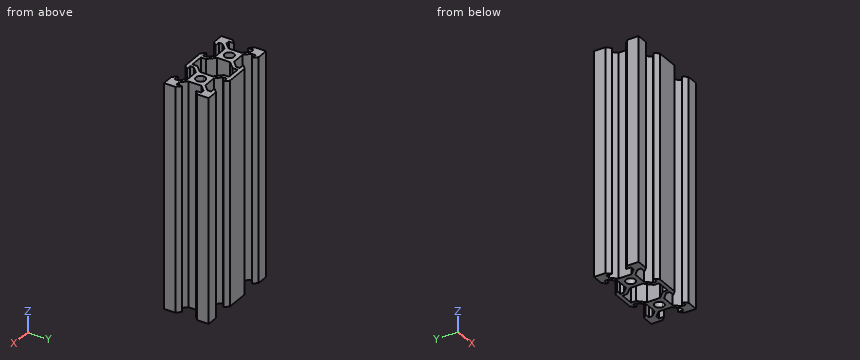
```python
from build123d import *

# Parameters (mm, degrees)
PAD_DEPTH            = 100
PAD_MIRRORED_2_DEPTH = 100


with BuildPart() as part:
    # Sketch → Pad (new body)
    with BuildSketch(Plane.XY):
        with BuildLine():
            Line((0, 10), (5.1, 10))
            Line((5.1, 10), (6.9, 8.2))
            Line((6.9, 8.2), (4.5, 8.2))
            Line((4.5, 8.2), (4.5, 6.56066))
            Line((4.5, 6.56066), (7.06066, 4))
            Line((7.06066, 4), (12.93934, 4))
            Line((12.93934, 4), (15.5, 6.56066))
            Line((15.5, 6.56066), (15.5, 8.2))
            Line((15.5, 8.2), (13.1, 8.2))
            Line((13.1, 8.2), (14.9, 10))
            Line((14.9, 10), (20, 10))
            Line((20, 10), (20, 4.9))
            Line((20, 4.9), (18.2, 3.1))
            Line((18.2, 3.1), (18.2, 5.5))
            Line((18.2, 5.5), (16.56066, 5.5))
            Line((16.56066, 5.5), (14, 2.93934))
            Line((14, 2.93934), (14, 0))
            Line((14, 0), (12.1, 0))
            ThreePointArc((12.1, 0), (10, 2.1), (7.9, 0))
            Line((7.9, 0), (6, 0))
            Line((6, 0), (6, 2.93934))
            Line((6, 2.93934), (3, 5.93934))
            Line((3, 5.93934), (3, 8.2))
            Line((3, 8.2), (0, 8.2))
            Line((0, 10), (0, 8.2))
        make_face()
    pad = extrude(amount=PAD_DEPTH)

    # Sketch Mirrored 2 → Pad Mirrored 2 (add)
    with BuildSketch(Plane(origin=(0, 0, 0), x_dir=(-1, 0, 0), z_dir=(0, 0, -1))):
        with BuildLine():
            Line((0, 10), (5.1, 10))
            Line((5.1, 10), (6.9, 8.2))
            Line((6.9, 8.2), (4.5, 8.2))
            Line((4.5, 8.2), (4.5, 6.56066))
            Line((4.5, 6.56066), (7.06066, 4))
            Line((7.06066, 4), (12.93934, 4))
            Line((12.93934, 4), (15.5, 6.56066))
            Line((15.5, 6.56066), (15.5, 8.2))
            Line((15.5, 8.2), (13.1, 8.2))
            Line((13.1, 8.2), (14.9, 10))
            Line((14.9, 10), (20, 10))
            Line((20, 10), (20, 4.9))
            Line((20, 4.9), (18.2, 3.1))
            Line((18.2, 3.1), (18.2, 5.5))
            Line((18.2, 5.5), (16.56066, 5.5))
            Line((16.56066, 5.5), (14, 2.93934))
            Line((14, 2.93934), (14, 0))
            Line((14, 0), (12.1, 0))
            ThreePointArc((12.1, 0), (10, 2.1), (7.9, 0))
            Line((7.9, 0), (6, 0))
            Line((6, 0), (6, 2.93934))
            Line((6, 2.93934), (3, 5.93934))
            Line((3, 5.93934), (3, 8.2))
            Line((3, 8.2), (0, 8.2))
            Line((0, 10), (0, 8.2))
        make_face()
    pad_mirrored_2 = extrude(amount=-PAD_MIRRORED_2_DEPTH)

    # Mirrored001: Pad, Pad Mirrored 2 across Sketch H_Axis
    add(pad.mirror(Plane.ZX))
    add(pad_mirrored_2.mirror(Plane.ZX))


solid = part.part
```
For this review, take the finished solid that the model builds, in its own axes (mm). Give positions to 0.01 mm unless a question says otherwise; leave off trailing zeros. Write each loop counter-clockwise with the first axis right and the second up, starting at its lowest first coordinate (ties: lowest second). Pieces come first, ordered by that corner, then holes. Notation, with made-up numbers: M 26.5,79.25 L 30.5,79.25 A26 ccw 30.5,114.25 Z; hole C -11,35.5 d7. An arc over 180 degrees is marked long. Answer as a JSON object with one key per item and string values. Group by question number.
Item 1: For probe 1 along X at (y, z) = (0, 56.5); probe 2 along X at (y, z) = (7.5, 46.5); probe 3 along Y at (x, z) = (1, 83), list the stretches that pass through material, from the lowest coordinate up. Write a range as [from, to].
Item 2: Consider section B-B on z = 73. Count the separate pieces of the cut face and the enclosed holes in it, plus the area to 3 significant figures.
Item 3: Consider section A-A on x = 10. Write out the cut boundary in (y, z).
Item 4: For pin 1 Ø1.2 at (x, z) = (-14, 42) entering from +Y; pin 2 Ø1.8 at (x, z) = (9, 50.5) entering from +Y; pin 3 Ø1.5 at (y, z) = (0.5, 37.5) entering from -X, all flat-tipped, find the tip position at first contact; note any pin that passes through.
Check result:
{
 "1": {"probe 1": "x = [-14, -12.1], [-7.9, -6], [6, 7.9], [12.1, 14]", "probe 2": "x = [-20, -15.5], [-4.5, -3], [3, 4.5], [15.5, 20]", "probe 3": "y = [-10, -8.2], [8.2, 10]"},
 "2": {"separate pieces": "1", "enclosed holes": "3", "area": "296 mm^2"},
 "3": {"outline": "M -4,0 L -2.1,0 L -2.1,100 L -4,100 Z; M 2.1,0 L 4,0 L 4,100 L 2.1,100 Z"},
 "4": {"pin 1": "stops at y = 9.7", "pin 2": "stops at y = 4", "pin 3": "stops at x = -14"}
}
